For this review, take the finished solid that the model builds, in its own axes (mm). A direction names the side the tool comes from. Round coordinates to 2 decimals unless told otherwise and drop trailing zeros. Loops run counter-clockwise (first coordinate to the right, second up) from the corner with the lowest first, then second, coordinate; pieces in that order, holes last.
1) Take a section at C-C (z = 3.75). State the section outline as (x, y) points, then the cut area to 3 significant figures.
2) Mouldability with a two-part tool opening along Z and no side actions: class faces 6 (the flat face through (-7.42, -12.68, 3.7)), 7 (the flat face through (0, -13.2, 4)), 8 (the cylindrical face through (1.09, 19.78, 6.93)) as pulls with the +Z half, pulls with the -Z half, needs draft (parallel to the pull), parting line crosses it, or undercut.
3) Take a section at A-A (y = 6.5). State the section outline as (x, z) points, then the cut area to 3 significant figures.
4) Tool access review of faces 1 (the flat face through (-1.7, 19, 3)), 2 (the flat face through (-0.5, 15, 2)), 3 (the flat face through (1.7, 19, 4)), 4 (the cylindrical face through (-0.8, 12.2, 3.7)), 5 (the cylindrical face through (-1.108, 15.812, 1.976)): name each direction out of +Z, -Z, +X, -X, +Y, -Y from which nothing blocks a thin tool from reaching the whole face with its end or side.
5) Take a section at D-D (y = 18). State the section outline as (x, z) points, then the cut area to 3 significant figures.
6) Insertion check: pin 1 (1.9 mm diameter, centred on y = 15.5, z = 4, fed in from -X); pin 2 (14.5 mm diameter, centred on x = 0, y = 0, fed in from +Z); pin 3 (1.9 mm diameter, centred on y = 17.5, z = 2.5, fed in from +X); pin 4 (1.8 mm diameter, centred on x = -0.5, z = 2.5, fed in from -Y). Each pin has a flat end and moves straight along its axis. Give the tip position at first contact, or say it passes through.
7) Wall thickness on L1, parallel to Z at x = 0, y = -15.05; L2, parallel to X at y = 15.5, z = 7; L3, parallel to X at y = -6, z = 6.25: over which ranges is each line inside the solid? List them lowest first.
8) Take a section at B-B (x = 9.5). State the section outline as (y, z) points.
```python
from build123d import *

# Parameters (mm, degrees)
F1_DEPTH    = 7.5
F2_R        = 3
F3_DEPTH    = 5
F4_R        = 2
F5_DEPTH    = 1.2
F6_R        = 1.7
F7_DEPTH    = 1.2
F8_T1_DEPTH = 7.5
F8_T3_DEPTH = 12.1179638093
F9_R        = 2


# Not quite as in the source:
# - a fillet or chamfer that OpenCascade refuses, or shapes differently, is made with other operations: its cross-section is extruded or revolved along the edge and cut away or added


with BuildPart() as f1:
    # F0 (on Top) → F1 (new body)
    with BuildSketch(Plane.XY):
        with BuildLine():
            ThreePointArc((10.9918685576, -7.3088182167), (0, -13.1999999285), (-10.9918685576, -7.3088182167))
            Line((-10.9918685576, -7.3088182167), (-3.75, -18.1999999285))
            Line((-3.75, -18.1999999285), (3.75, -18.1999999285))
            Line((3.75, -18.1999999285), (10.9918685576, -7.3088182167))
        make_face()
        with BuildLine():
            ThreePointArc((1.7, 11.8789730196), (9.0664215653, 7.8612976028), (12, 0))
            ThreePointArc((12, 0), (-7.8612976028, -9.0664215653), (-1.7, 11.8789730196))
            Line((-1.7, 11.8789730196), (-1.7, 13.0900725022))
            ThreePointArc((-1.7, 13.0900725022), (-12.0124754947, 5.4717849557), (-10.9918685576, -7.3088182167))
            ThreePointArc((-10.9918685576, -7.3088182167), (0, -13.1999999285), (10.9918685576, -7.3088182167))
            ThreePointArc((10.9918685576, -7.3088182167), (12.6359143374, -3.8175472451), (13.1999999285, 0))
            ThreePointArc((13.1999999285, 0), (9.9166526104, 8.7120605552), (1.7, 13.0900725022))
            Line((1.7, 13.0900725022), (1.7, 11.8789730196))
        make_face()
        with BuildLine():
            ThreePointArc((0.5, 13.1905268322), (1.1011461157, 13.1539908523), (1.7, 13.0900725022))
            Line((1.7, 13.0900725022), (1.7, 20.3789730196))
            Line((1.7, 20.3789730196), (0.5, 20.3789730196))
            Line((0.5, 20.3789730196), (0.5, 13.1905268322))
        make_face()
        with BuildLine():
            Line((-1.7, 20.3789730196), (-1.7, 13.0900725022))
            ThreePointArc((-1.7, 13.0900725022), (-1.1011461157, 13.1539908523), (-0.5, 13.1905268322))
            Line((-0.5, 13.1905268322), (-0.5, 20.3789730196))
            Line((-0.5, 20.3789730196), (-1.7, 20.3789730196))
        make_face()
        with BuildLine():
            Line((-1.7, 13.0900725022), (-1.7, 11.8789730196))
            ThreePointArc((-1.7, 11.8789730196), (-1.1013893091, 11.9493490028), (-0.5, 11.9895788083))
            Line((-0.5, 11.9895788083), (-0.5, 13.1905268322))
            ThreePointArc((-0.5, 13.1905268322), (-1.1011461157, 13.1539908523), (-1.7, 13.0900725022))
        make_face()
        with BuildLine():
            ThreePointArc((0.5, 11.9895788083), (1.1013893091, 11.9493490028), (1.7, 11.8789730196))
            Line((1.7, 11.8789730196), (1.7, 13.0900725022))
            ThreePointArc((1.7, 13.0900725022), (1.1011461157, 13.1539908523), (0.5, 13.1905268322))
            Line((0.5, 13.1905268322), (0.5, 11.9895788083))
        make_face()
    extrude(amount=F1_DEPTH)

    # F2 (on face) → F3 (cut)
    with BuildSketch(Plane.XZ.offset(18.1999999285)):
        with Locations((0, 3.75)):
            Circle(F2_R)
    extrude(amount=-F3_DEPTH, mode=Mode.SUBTRACT)

    # F4 (on face) → F5 (cut, through all)
    with BuildSketch(Plane(origin=(-1.7, 0, 0), x_dir=(0, -1, 0), z_dir=(-1, 0, 0))):
        with Locations((-16.7345227609, 3.75)):
            Circle(F4_R)
    extrude(amount=-F5_DEPTH, mode=Mode.SUBTRACT)

    # F6 (on face) → F7 (cut, through all)
    with BuildSketch(Plane.YZ.offset(1.7)):
        with Locations((16.7345227609, 3.75)):
            Circle(F6_R)
    extrude(amount=-F7_DEPTH, mode=Mode.SUBTRACT)

    # F8: fillet of radius 1 on 5 edges, made by hand

    # F8_s2 → F8_t1 (join)
    with BuildSketch(Plane.XY):
        with BuildLine():
            ThreePointArc((-2.509859154, 12.9591899878), (-1.9285919219, 13.3046060392), (-1.7, 13.9409468103))
            Line((-1.7, 13.9409468103), (-1.7, 13.0900725022))
            ThreePointArc((-1.7, 13.0900725022), (-2.1059466, 13.0309242585), (-2.509859154, 12.9591899878))
        make_face()
        with BuildLine():
            ThreePointArc((2.509859154, 12.9591899878), (1.9285919219, 13.3046060392), (1.7, 13.9409468103))
            Line((1.7, 13.9409468103), (1.7, 13.0900725022))
            ThreePointArc((1.7, 13.0900725022), (2.1059466, 13.0309242585), (2.509859154, 12.9591899878))
        make_face()
    extrude(amount=F8_T1_DEPTH)

    # F8_s4 → F8_t3 (cut)
    with BuildSketch(Plane.XY.offset(-2.3089819047)):
        with BuildLine():
            ThreePointArc((-1.3846153846, 11.9198506801), (-0.7532120062, 12.2481093984), (-0.5, 12.9131715701))
            Line((-0.5, 12.9131715701), (-0.5, 11.9895788083))
            ThreePointArc((-0.5, 11.9895788083), (-0.9429524325, 11.9628943283), (-1.3846153846, 11.9198506801))
        make_face()
        with BuildLine():
            ThreePointArc((0.5, 12.9131715701), (0.7532120062, 12.2481093984), (1.3846153846, 11.9198506801))
            ThreePointArc((1.3846153846, 11.9198506801), (0.9429524325, 11.9628943283), (0.5, 11.9895788083))
            Line((0.5, 11.9895788083), (0.5, 12.9131715701))
        make_face()
    extrude(amount=F8_T3_DEPTH, mode=Mode.SUBTRACT)

    # F8_s5 → F8_t6 (revolve, cut)
    with BuildSketch(Plane.XY.offset(3.75)):
        with BuildLine():
            ThreePointArc((4, -18.1999999285), (3.2928932188, -17.9071067097), (3, -17.1999999285))
            Line((3, -17.1999999285), (3, -18.1999999285))
            Line((3, -18.1999999285), (4, -18.1999999285))
        make_face()
    revolve(axis=Axis((0, -18.1999999285, 3.75), (0, -1, 0)), mode=Mode.SUBTRACT)

    # F9
    f9_edges = [f1.edges().sort_by_distance(p)[0] for p in [
        (-1.1, 20.378973, 7.5),
        (1.1, 20.378973, 7.5),
        (1.1, 20.378973, 0),
        (-1.1, 20.378973, 0),
    ]]
    fillet(f9_edges, radius=F9_R)


solid = f1.part
```
Response:
1. outline: (-10.99, -7.31) - (-3.77, -18.17) arc R1 ccw to (-3, -17.2) - (-3, -13.2) - (3, -13.2) - (3, -17.2) arc R1 ccw to (3.77, -18.17) - (10.99, -7.31) arc R13.2 ccw to (2.51, 12.96) arc R1 cw to (1.7, 13.94) - (1.7, 15.03) - (0.5, 15.03) - (0.5, 12.91) arc R1 ccw to (1.38, 11.92) arc R12 cw (long way) to (-1.38, 11.92) arc R1 ccw to (-0.5, 12.91) - (-0.5, 14.73) - (-1.7, 14.73) - (-1.7, 13.94) arc R1 cw to (-2.51, 12.96) arc R13.2 ccw to start; (-1.7, 18.73) - (-0.5, 18.73) - (-0.5, 20.38) - (-1.7, 20.38) - close; (0.5, 18.43) - (1.7, 18.43) - (1.7, 20.38) - (0.5, 20.38) - close
1. area: 141 mm2
2. face 6: needs draft
2. face 7: undercut
2. face 8: pulls with the +Z half
3. outline: (-11.49, 0) - (-10.09, 0) - (-10.09, 7.5) - (-11.49, 7.5) - close; (10.09, 0) - (11.49, 0) - (11.49, 7.5) - (10.09, 7.5) - close
3. area: 21.0 mm2
4. face 1: +Z, -Z, -X, +Y
4. face 2: +Z, -Z, +Y
4. face 3: +Z, -Z, +X, +Y
4. face 4: +Z, -Z
4. face 5: -X
5. outline: (-1.7, 0) - (-0.5, 0) - (-0.5, 2.2) - (-1.7, 2.2) - close; (-1.7, 5.3) - (-0.5, 5.3) - (-0.5, 7.5) - (-1.7, 7.5) - close; (0.5, 0) - (1.7, 0) - (1.7, 2.61) - (0.5, 2.61) - close; (0.5, 4.89) - (1.7, 4.89) - (1.7, 7.5) - (0.5, 7.5) - close
5. area: 11.6 mm2
6. pin 1: stops at x = -1.7
6. pin 2: passes through
6. pin 3: stops at x = 1.7
6. pin 4: stops at y = -13.2
7. L1: z = 0 to 0.75, 6.75 to 7.5
7. L2: x = -1.7 to -0.5, 0.5 to 1.7
7. L3: x = -11.76 to -10.39, 10.39 to 11.76
8. outline: (-9.55, 0) - (-7.33, 0) - (-7.33, 7.5) - (-9.55, 7.5) - close; (7.33, 0) - (9.16, 0) - (9.16, 7.5) - (7.33, 7.5) - close
